Geometry check sheet. Reference: drawing and pictorial views, mm from the part's lowest x, y, z. A direction names the side the tool comes from. Give positions to 0.01 mm unless a question says otherwise; leave off trailing zeros. Write each loop counter-clockwise with the first axis right and the second up, starting at its lowest first coordinate (ties: lowest second). Pieces come first, ordered by that corner, then holes. Notation, with made-up numbers: (50.5, 54.5) -> (60.5, 54.5) arc R16 cw to (60.5, 61.5) -> close; hole circle Ø1 at (1.5, -3.75). An arc over 180 degrees is marked (long way). Use a Markdown table: item, result. Add a question column.
1. Scan lines: probe 1 along Y at (x, z) = (17, 10.2); probe 2 along X at (y, z) = (3.1, 5.89); probe 3 along Y at (x, z) = (16.5, 5.25). Record each from-to range of solid material in increasing order. Write a range as [from, to].
2. Gauge pin test, flat ends, axial feed: P1, Ø1, axis at x = 28.5, z = 4, coming from the +Y side; P2, Ø2, axis at x = 26.5, z = 17, coming from the +Y side; P3, Ø3.5, axis at x = 28.935, z = 24.11, coming from the -Y side; P4, Ø5, axis at x = 5, y = 17.5, coming from the -Z side. Record the tip position at first contact, or that the pin passes through.
3. Cross-section at D-D (z = 25.25). Enter the section's corners in (x, y), then the cut area to 3 significant figures.
4. Cross-section at C-C (x = 17). Count the separate pieces of the cut face and the enclosed holes in it, then the cut area to 3 significant figures.
5. Cross-section at B-B (z = 5.89). Enter the section's corners in (x, y), then the cut area to 3 significant figures.
6. Release check for a two-part mould opening along Y. For the marked faces 5, 6 and 7 record: released by +Y, released by -Y, zero draft, split by the parting line, or undercut.
7. Set-up check for the marked faces 1, 2, 3 and 4: record each of +Z, -Z, +X, -X, +Y, -Y from which the full face is reachable in a straight line by a thin tool's end or side.
8. Cross-section at A-A (y = 59.72). Enter the section's corners in (x, z), then the cut area to 3 significant figures.
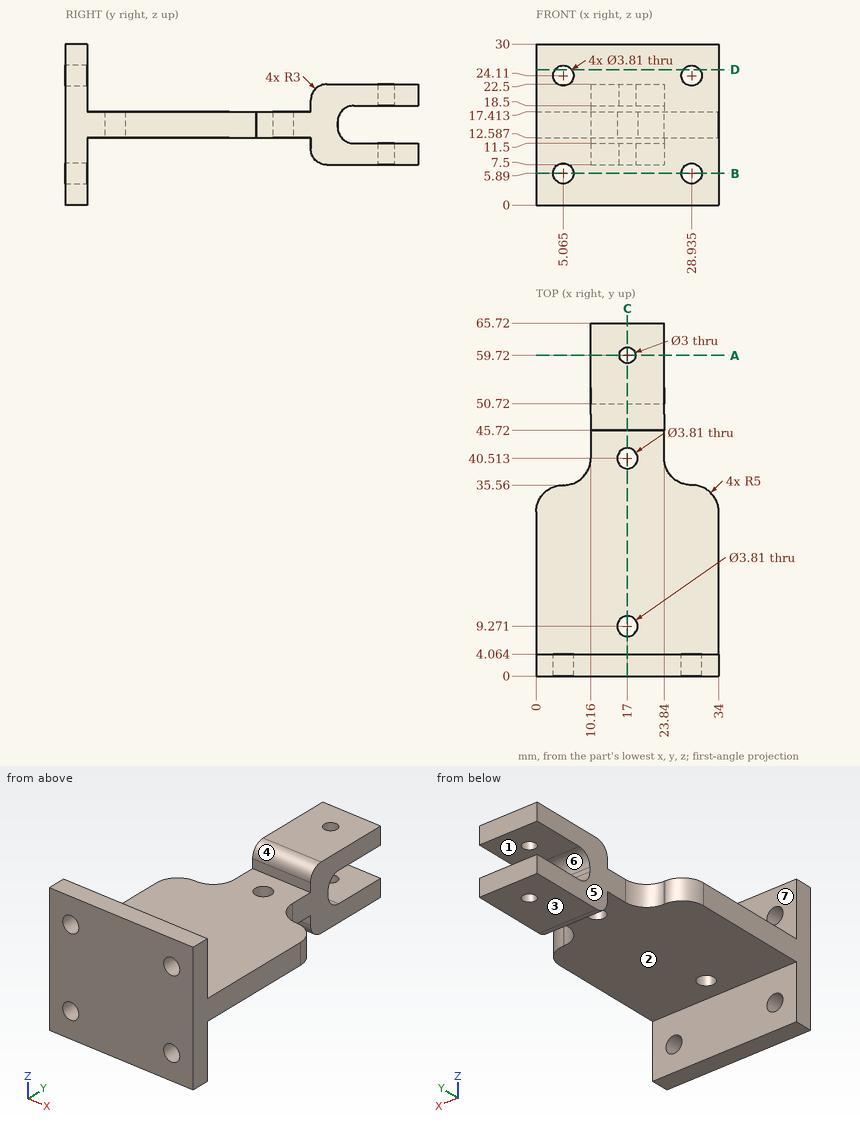
Worked answers:
| question | item | result |
|---|---|---|
| 1 | probe 1 | y = [0, 4.06], [45.74, 58.22], [61.22, 65.72] |
| 1 | probe 2 | x = [0, 3.16], [6.97, 27.03], [30.84, 34] |
| 1 | probe 3 | y = [0, 4.06] |
| 2 | P1 | stops at y = 4.06 |
| 2 | P2 | stops at y = 36.84 |
| 2 | P3 | passes through |
| 2 | P4 | stops at z = 12.59 |
| 3 | outline | (0, 0) -> (3.54, 0) -> (3.54, 4.06) -> (0, 4.06) -> close; (6.59, 0) -> (27.41, 0) -> (27.41, 4.06) -> (6.59, 4.06) -> close; (30.46, 0) -> (34, 0) -> (34, 4.06) -> (30.46, 4.06) -> close |
| 3 | area | 113 mm² |
| 4 | separate pieces | 5 |
| 4 | enclosed holes | 0 |
| 4 | area | 457 mm² |
| 5 | outline | (0, 0) -> (3.16, 0) -> (3.16, 4.06) -> (0, 4.06) -> close; (6.97, 0) -> (27.03, 0) -> (27.03, 4.06) -> (6.97, 4.06) -> close; (30.84, 0) -> (34, 0) -> (34, 4.06) -> (30.84, 4.06) -> close |
| 5 | area | 107 mm² |
| 6 | face 5 | zero draft |
| 6 | face 6 | released by +Y |
| 6 | face 7 | undercut |
| 7 | face 1 | +X, -X, +Y |
| 7 | face 2 | -Z, +X, -X |
| 7 | face 3 | -Z, +X, -X, +Y |
| 7 | face 4 | +Z, +X, -X |
| 8 | outline | (10.16, 7.5) -> (15.5, 7.5) -> (15.5, 11.5) -> (10.16, 11.5) -> close; (10.16, 18.5) -> (15.5, 18.5) -> (15.5, 22.5) -> (10.16, 22.5) -> close; (18.5, 7.5) -> (23.84, 7.5) -> (23.84, 11.5) -> (18.5, 11.5) -> close; (18.5, 18.5) -> (23.84, 18.5) -> (23.84, 22.5) -> (18.5, 22.5) -> close |
| 8 | area | 85.4 mm² |
